from build123d import *

# Parameters (mm, degrees)
SKETCH1_W               = 76
SKETCH1_H               = 63
BOSS_EXTRUDE1_DEPTH     = 2
SKETCH2_W               = 69.6
SKETCH2_H               = 56.6
BOSS_EXTRUDE2_DEPTH     = 1
SKETCH3_W               = 69.8
SKETCH3_H               = 3.2
BOSS_EXTRUDE3_DEPTH     = 32
BOSS_EXTRUDE4_DEPTH     = 3.5
BOSS_EXTRUDE5_DEPTH     = 3.5
BOSS_EXTRUDE6_DEPTH     = 3.5
CUT_EXTRUDE1_DEPTH      = 7
CHAMFER1_SIZE           = 2
FILLET1_SIZE            = 2
CUT_EXTRUDE2_DEPTH      = 81.23091686
CUT_EXTRUDE2_DEPTH_BACK = 3.2
SKETCH8_R               = 7
SKETCH8_W               = 12
SKETCH8_H               = 9
SKETCH9_W               = 17.861030929
SKETCH9_H               = 28
CUT_EXTRUDE3_DEPTH      = 1
SKETCH10_W              = 69.6
SKETCH10_H              = 8
CUT_EXTRUDE4_DEPTH      = 2
CHAMFER2_SIZE2          = 1
CHAMFER2_SIZE           = 1.732050808
CUT_EXTRUDE5_DEPTH      = 3.2


# Some blends are built 0.0001 mm under size
with BuildPart() as part:
    # Sketch1 → Boss-Extrude1 (new body)
    with BuildSketch(Plane(origin=(0, 0, 0), x_dir=(1, 0, 0), z_dir=(0, 1, 0))):
        Rectangle(SKETCH1_W, SKETCH1_H)
    extrude(amount=BOSS_EXTRUDE1_DEPTH)

    # Sketch2 → Boss-Extrude2 (add)
    with BuildSketch(Plane(origin=(0, 0, 0), x_dir=(1, 0, 0), z_dir=(0, 1, 0))):
        Rectangle(SKETCH2_W, SKETCH2_H)
    extrude(amount=-BOSS_EXTRUDE2_DEPTH)

    # Sketch3 → Boss-Extrude3 (add)
    with BuildSketch(Plane.XZ):
        with Locations((0, -29.9)):
            Rectangle(SKETCH3_W, SKETCH3_H)
    extrude(amount=BOSS_EXTRUDE3_DEPTH)

    # Sketch4 → Boss-Extrude4 (add, symmetric)
    with BuildSketch(Plane.XY.offset(-1.5)):
        Polygon((-34.8, 0), (-36, -1.5), (-34.8, -3), (-33.3, -3), (-33.3, 0), align=None)
        Polygon((33.3, 0), (34.8, 0), (36, -1.5), (34.8, -3), (33.3, -3), align=None)
    extrude(amount=BOSS_EXTRUDE4_DEPTH, both=True)

    # Sketch5 → Boss-Extrude5 (add, symmetric)
    with BuildSketch(Plane(origin=(0, 0, 0), x_dir=(0, 0, -1), z_dir=(1, 0, 0))):
        Polygon((-28.3, 0), (-29.5, -1.5), (-28.3, -3), (-27.3, -3), (-27.3, 0), align=None)
    extrude(amount=BOSS_EXTRUDE5_DEPTH, both=True)

    # Sketch6 → Boss-Extrude6 (add, symmetric)
    with BuildSketch(Plane(origin=(0, -16, 0), x_dir=(-1, 0, 0), z_dir=(0, -1, 0))):
        Polygon((-34.9, 31.5), (-36, 30), (-34.9, 28.3), align=None)
        Polygon((34.9, 28.3), (34.9, 31.5), (36, 30), align=None)
    extrude(amount=BOSS_EXTRUDE6_DEPTH, both=True)

    # Sketch7 → Cut-Extrude1 (cut)
    with BuildSketch(Plane.XZ.offset(1)):
        with BuildLine():
            Line((-26.822034097, -5.879323383), (-26.822034097, -15.516493675))
            ThreePointArc((-26.822034097, -15.516493675), (-24.522034097, -17.816493675), (-22.222034097, -15.516493675))
            Line((-22.222034097, -15.516493675), (-22.222034097, -5.879323383))
            ThreePointArc((-22.222034097, -5.879323383), (-24.522034097, 1.393290251), (-26.822034097, -5.879323383))
        make_face()
        with BuildLine():
            Line((22.222034097, -5.879323383), (22.222034097, -15.516493675))
            ThreePointArc((22.222034097, -15.516493675), (24.522034097, -17.816493675), (26.822034097, -15.516493675))
            Line((26.822034097, -15.516493675), (26.822034097, -5.879323383))
            ThreePointArc((26.822034097, -5.879323383), (24.522034097, 1.393290251), (22.222034097, -5.879323383))
        make_face()
    extrude(amount=-CUT_EXTRUDE1_DEPTH, mode=Mode.SUBTRACT)

    # Chamfer1
    chamfer1_edges = [part.edges().sort_by_distance(p)[0] for p in [
        (-24.522034097, -1, 1.393290251),
        (-26.822034097, -1, -10.697908529),
        (-24.522034097, -1, -17.816493675),
        (-22.222034097, -1, -10.697908529),
        (24.522034097, -1, -17.816493675),
        (26.822034097, -1, -10.697908529),
        (24.522034097, -1, 1.393290251),
        (22.222034097, -1, -10.697908529),
    ]]
    chamfer(chamfer1_edges, length=CHAMFER1_SIZE)

    # Fillet1
    # a fillet whose section is not a circle: 2 mm, written as the material it takes off along each edge
    with BuildSketch(Plane(origin=(38, -5, 31.5), x_dir=(0, 0, -1), z_dir=(0, 1, 0)), Plane(origin=(38, -5, -31.5), x_dir=(-1, 0, 0), z_dir=(0, 1, 0))) as fillet1_piece_1:
        with BuildLine():
            add(Edge.make_bspline([(FILLET1_SIZE, 0), (FILLET1_SIZE * 0.831801948466, 0), (FILLET1_SIZE * 0.663603896932, 0), (FILLET1_SIZE * 0.292893218813, FILLET1_SIZE * 0.0716919198361), (FILLET1_SIZE * 0.0716919198361, FILLET1_SIZE * 0.292893218813), (0, FILLET1_SIZE * 0.663603896932), (0, FILLET1_SIZE * 0.831801948466), (0, FILLET1_SIZE)], knots=[0, 0, 0, 0, 0, 0, 0.5, 0.5, 1, 1, 1, 1, 1, 1], degree=5))
            Line((0, FILLET1_SIZE), (0, 0))
            Line((0, 0), (FILLET1_SIZE, 0))
        make_face()
    extrude(amount=12, mode=Mode.SUBTRACT)
    with BuildSketch(Plane(origin=(-38, -5, 31.5), x_dir=(0, 0, -1), z_dir=(0, 1, 0)), Plane(origin=(-38, -5, -31.5), x_dir=(1, 0, 0), z_dir=(0, 1, 0))) as fillet1_piece_2:
        with BuildLine():
            add(Edge.make_bspline([(FILLET1_SIZE, 0), (FILLET1_SIZE * 0.831801948466, 0), (FILLET1_SIZE * 0.663603896932, 0), (FILLET1_SIZE * 0.292893218813, -FILLET1_SIZE * 0.0716919198361), (FILLET1_SIZE * 0.0716919198361, -FILLET1_SIZE * 0.292893218813), (0, -FILLET1_SIZE * 0.663603896932), (0, -FILLET1_SIZE * 0.831801948466), (0, -FILLET1_SIZE)], knots=[0, 0, 0, 0, 0, 0, 0.5, 0.5, 1, 1, 1, 1, 1, 1], degree=5))
            Line((0, -FILLET1_SIZE), (0, 0))
            Line((0, 0), (FILLET1_SIZE, 0))
        make_face()
    extrude(amount=12, mode=Mode.SUBTRACT)

    # Sketch8 → Cut-Extrude2 (cut, two sides: drawn at the far end of the back side and taken through both)
    with BuildSketch(Plane(origin=(0, 0, -31.5), x_dir=(-1, 0, 0), z_dir=(0, 0, -1)).offset(-CUT_EXTRUDE2_DEPTH_BACK)):
        with Locations((14.4, -21.8)):
            Circle(SKETCH8_R)
        with BuildLine():
            Line((-19.95069293, -22), (-11.95069293, -22))
            ThreePointArc((-11.95069293, -22), (-6.95069293, -27), (-11.95069293, -32))
            Line((-11.95069293, -32), (-19.95069293, -32))
            ThreePointArc((-19.95069293, -32), (-24.95069293, -27), (-19.95069293, -22))
        make_face()
        with Locations((-21.4, -4)):
            Rectangle(SKETCH8_W, SKETCH8_H)
    extrude(amount=CUT_EXTRUDE2_DEPTH + CUT_EXTRUDE2_DEPTH_BACK, mode=Mode.SUBTRACT)

    # Sketch9 → Cut-Extrude3 (cut)
    with BuildSketch(Plane.XZ.offset(1)):
        with Locations((24.330515464, -14.3)):
            Rectangle(SKETCH9_W, SKETCH9_H)
    extrude(amount=-CUT_EXTRUDE3_DEPTH, mode=Mode.SUBTRACT)

    # Sketch10 → Cut-Extrude4 (cut)
    with BuildSketch(Plane.XZ.offset(1)):
        with Locations((0, 23.3)):
            Rectangle(SKETCH10_W, SKETCH10_H)
    extrude(amount=-CUT_EXTRUDE4_DEPTH, mode=Mode.SUBTRACT)

    # Chamfer2
    chamfer2_edges = [part.edges().sort_by_distance(p)[0] for p in [
        (0, -3, 27.3),
    ]]
    chamfer2_side = [part.faces().sort_by_distance(p)[0] for p in [
        (0, -2.98, 27.3),
    ]]
    chamfer(chamfer2_edges, length=CHAMFER2_SIZE - 0.0001, length2=CHAMFER2_SIZE2 - 0.0001, reference=chamfer2_side[0])  # a hair under: the kernel refuses the full size

    # Sketch11 → Cut-Extrude5 (cut)
    with BuildSketch(Plane(origin=(0, 0, -31.5), x_dir=(-1, 0, 0), z_dir=(0, 0, -1))):
        Polygon((-24.798914111, -28.222600255), (-24.798914111, -36.274254695), (17.416877144, -36.274254695), (17.416877144, -28.116522168), (7.402857726, -22), (-13.082910041, -22), (-13.082910041, -28.222600255), align=None)
    extrude(amount=-CUT_EXTRUDE5_DEPTH, mode=Mode.SUBTRACT)


solid = part.part
Input: part model. Units: mm. Frame: model coordinates. A direction names the side the tool comes from. Coordinates: 2 decimals unless noted, no trailing zeros. Loops run counter-clockwise (first coordinate to the right, second up) from the corner with the lowest first, then second, coordinate; pieces in that order, holes last.
(1) First-contact query: pin 1 Ø0.5 at (y, z) = (-0.5, 28) entering from +X; pin 2 Ø1 at (x, z) = (13.5, 15.5) entering from -Y; pin 3 Ø0.8 at (x, z) = (34, -1) entering from -Y. Flat tips, straight axial feed; report the tip coordinate or a pass-through.
(2) Material intervals for probe 1 along Y at (x, z) = (-21.5, -24); probe 2 along Z at (x, y) = (-25, -21); probe 3 along Y at (x, z) = (-14.4, -29.2), sorted ascending.
(3) Section D-D on z = 14. Return the cut outline in (x, y), then the cut area to 3 significant figures.
(4) Pull-direction query (Y, two-part tool) for faces 5 (the face through (-21.236, 0.014, -10.765)), 6 (the face through (24.471, 1.493, -17.816)), 7 (the face through (34.9, -6, -30)); classes: released by +Y, released by -Y, zero draft, split by the parting line, or undercut.
(5) Section B-B on x = -14.4. Return the cut outline in (y, z), then the cut area to 3 significant figures.
(6) Section A-A on z = -8. Return the cut outline in (x, y).
(7) Section C-C on y = -26. Return the cut outline in (x, z).
(8) Set-up query: faces 1 (the face through (15.4, -0.7, -22.9)), 2 (the face through (-24.38, 1.49, 1.39)), 3 (the face through (-33.3, -2, -2)), 4 (the face through (-24.58, 0.681, -18.135)). Return all of +Z, -Z, +X, -X, +Y, -Y with unobstructed straight access to the full face (end or side cutting, diameter ignored); none if empty.
Data:
1. pin 1: stops at x = 34.8
1. pin 2: stops at y = -1
1. pin 3: stops at y = -3
2. probe 1: y = -1 to 2
2. probe 2: z = -31.5 to -28.3
2. probe 3: y = -14.8 to 2
3. outline: (-38, 0) - (-34.8, 0) - (-34.8, -1) - (34.8, -1) - (34.8, 0) - (38, 0) - (38, 2) - (-38, 2) - close
3. area: 222 mm2
4. face 5: released by -Y
4. face 6: zero draft
4. face 7: undercut
5. outline: (-14.8, -31.5) - (2, -31.5) - (2, 31.5) - (0, 31.5) - (0, 28.3) - (-1, 28.3) - (-1, 27.3) - (1, 27.3) - (1, 19.3) - (-1, 19.3) - (-1, -28.3) - (-14.8, -28.3) - close
5. area: 214 mm2
6. outline: (-38, 0) - (-34.8, 0) - (-34.8, -1) - (-28.82, -1) - (-26.82, 1) - (-26.82, 2) - (-38, 2) - close; (-22.22, 1) - (-20.22, -1) - (15.4, -1) - (15.4, 0) - (21.22, 0) - (22.22, 1) - (22.22, 2) - (-22.22, 2) - close; (26.82, 1) - (27.82, 0) - (33.26, 0) - (33.26, -1) - (34.8, -1) - (34.8, 0) - (38, 0) - (38, 2) - (26.82, 2) - close
7. outline: (-34.9, -31.5) - (-20, -31.5) - (-20, -28.3) - (-34.9, -28.3) - close; (24.85, -31.5) - (34.9, -31.5) - (34.9, -28.3) - (24.85, -28.3) - close
8. face 1: -Z
8. face 2: +Y, -Y
8. face 3: +Z, -Y
8. face 4: -Y
